```python
from build123d import *

# Parameters (mm, degrees)
PAD_DEPTH       = 17.9
SKETCH001_R     = 1.5
POCKET_DEPTH    = 17.9
SKETCH003_R     = 0.5
POCKET001_DEPTH = 6
SKETCH004_R     = 0.5
POCKET002_DEPTH = 6
SKETCH005_R     = 1.1
POCKET003_DEPTH = 6.5
SKETCH006_R     = 1.1
POCKET004_DEPTH = 6.5


with BuildPart() as part:
    # Sketch → Pad (new body)
    with BuildSketch(Plane.XY):
        Polygon((0, 0), (18.5, 0), (18.5, 10.68097998), (9.25, 16.02146997), align=None)
    extrude(amount=PAD_DEPTH)

    # Sketch001 → Pocket (cut)
    with BuildSketch(Plane.XY.offset(17.9)):
        with Locations((12.3841632741, 7.15)):
            Circle(SKETCH001_R)
    extrude(amount=-POCKET_DEPTH, mode=Mode.SUBTRACT)

    # Sketch003 → Pocket001 (cut)
    with BuildSketch(Plane.XZ):
        with Locations((12.385, 17.9)):
            Circle(SKETCH003_R)
    extrude(amount=-POCKET001_DEPTH, mode=Mode.SUBTRACT)

    # Sketch004 → Pocket002 (cut)
    with BuildSketch(Plane(origin=(0, 0, 0), x_dir=(-0.5, -0.8660254038, 0), z_dir=(-0.8660254038, 0.5, 0))):
        with Locations((-12.385, 17.9)):
            Circle(SKETCH004_R)
    extrude(amount=-POCKET002_DEPTH, mode=Mode.SUBTRACT)

    # Sketch005 → Pocket003 (cut)
    with BuildSketch(Plane.XZ):
        with Locations((11, 15.2)):
            Circle(SKETCH005_R)
        with Locations((11, 2.5)):
            Circle(SKETCH005_R)
    extrude(amount=-POCKET003_DEPTH, mode=Mode.SUBTRACT)

    # Sketch006 → Pocket004 (cut)
    with BuildSketch(Plane(origin=(0, 0, 0), x_dir=(-0.5, -0.8660254038, 0), z_dir=(-0.8660254038, 0.5, 0))):
        with Locations((-11, 15.2)):
            Circle(SKETCH006_R)
        with Locations((-11, 2.5)):
            Circle(SKETCH006_R)
    extrude(amount=-POCKET004_DEPTH, mode=Mode.SUBTRACT)


solid = part.part
```
Geometry: final body of the model. Coordinates: model frame, mm. A direction names the side the tool comes from. Coordinates: 2 decimals unless noted, no trailing zeros. Order: outer loops, then holes, each group sorted by start corner. A loop starts at its lowest first (then second) coordinate and runs counter-clockwise, first axis right, second up. Notation, with made-up numbers: M 15,-37 L 45,-37 A14 ccw 45,-20 Z; hole C -36.5,-21 d10. An arc over 180 degrees is marked long. Answer in a Markdown table with one row per item. Add a question column.
Q1. Section query A-A on z = 8. Return the cut outline in (x, y), and give its area (3 significant figures).
Q2. Section query C-C on y = 4.25. Return the cut outline in (x, z) (3 decimals), and give its area (3 significant figures).
Q3. Mould query, pull axis Z, two halves, no side actions, for faces 4 (the flat face through (14, 8, 17.9)), 5 (the flat face through (4.69, 8.12, 8.82)), 6 (the cylindrical face through (9.9, 3.1, 2.5)). Classes: released by +Z, released by -Z, zero draft, split by the parting line, or undercut.
Q4. Section query B-B on z = 14.75. Return the cut outline in (x, y).
Q5. Contact query for flat-ended pins moving along their axis: P1, Ø2.5, axis at x = 12.38, y = 7.15, coming from the +Z side; P2, Ø1.5, axis at y = 6.5, z = 10, coming from the -X side; P3, Ø3, axis at x = 11, z = 15.2, coming from the +Y side; P4, Ø1, axis at y = 6.5, z = 8.5, coming from the -X side. Output: stop coordinate, or through.
Q6. Section query D-D on x = 15.5. Return the cut outline in (y, z).
Q7. Reachability of faces 1 (the cylindrical face through (12.4, 2.8, 17.4)), 2 (the flat face through (9, 6, 0)), 3 (the cylindrical face through (9.9, 3.1, 15.2)) from +Z, -Z, +X, -X, +Y, -Y: full face, straight path, thin tool, end or side. Return the list, or none.
Q8. Line query: L1, parallel to X at y = 7.15, z = 8.75; L2, parallel to Z at x = 10, y = 2; L3, parallel to X at y = 4.5, z = 2.5. Output: solid intervals per line, ascending.
Completed:
| question | item | result |
|---|---|---|
| 1 | outline | M 0,0 L 18.5,0 L 18.5,10.68 L 9.25,16.02 Z; hole C 12.38,7.15 d3 |
| 1 | area | 191 mm2 |
| 2 | outline | M 2.454,0 L 18.5,0 L 18.5,17.9 L 12.885,17.9 A0.5 cw 11.885,17.9 L 2.454,17.9 Z; hole C 11,2.5 d2.2; hole C 11,15.2 d2.2 |
| 2 | area | 279 mm2 |
| 3 | face 4 | released by +Z |
| 3 | face 5 | zero draft |
| 3 | face 6 | undercut |
| 4 | outline | M 0,0 L 10,0 L 10,5.77 L 5,8.66 Z; M 6,10.4 L 10.94,7.55 A1.5 cw long 12,5.7 L 12,0 L 18.5,0 L 18.5,10.68 L 9.25,16.02 Z |
| 5 | P1 | passes through |
| 5 | P2 | stops at x = 3.32 |
| 5 | P3 | stops at y = 15.88 |
| 5 | P4 | stops at x = 3.46 |
| 6 | outline | M 0,0 L 12.41,0 L 12.41,17.9 L 0,17.9 Z |
| 7 | face 1 | +Z, -Y |
| 7 | face 2 | -Z, +X, -X, +Y, -Y |
| 7 | face 3 | -Y |
| 8 | L1 | x = 4.13 to 10.88, 13.88 to 18.5 |
| 8 | L2 | z = 0 to 2.04, 2.96 to 14.74, 15.66 to 17.9 |
| 8 | L3 | x = 2.6 to 9.9, 12.1 to 18.5 |
